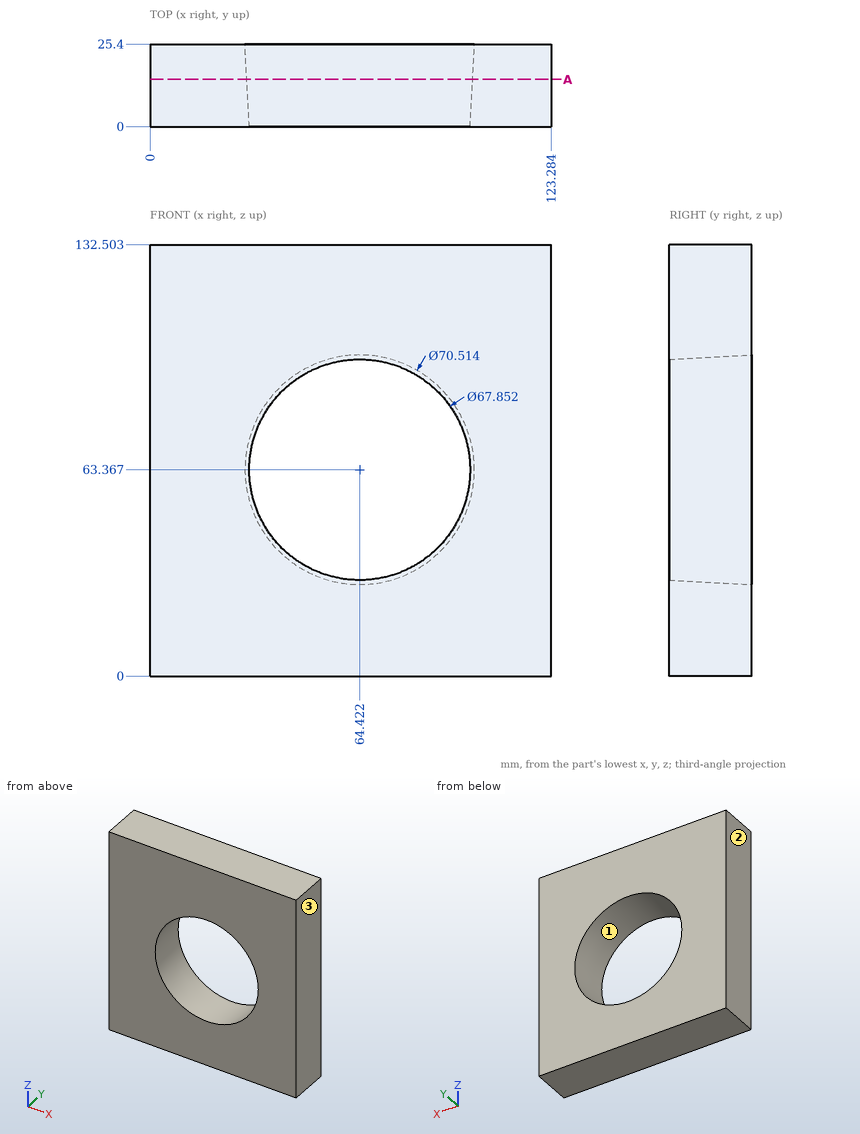
Geometry: see drawing. Coordinates: mm, zero at the bounding-box minimum. Round coordinates to 2 decimals unless told otherwise and drop trailing zeros. Write each loop counter-clockwise with the first axis right and the second up, starting at its lowest first coordinate (ties: lowest second). Pieces come first, ordered by that corner, then holes.
Item 1: Pin query (flat end, axial travel): P1, Ø3, axis at y = 13, z = 25, coming from the -X side. Return the tip coordinate at first contact, or that it passes through.
Item 2: Mould query, pull axis X, two halves, no side actions, for the marked faces 1, 2 and 3. Classes: +X half, -X half, draft (parallel to the pull), parting line (faces both ways), or undercut.
Item 3: Section query A-A (y = 14.5). Return loops of the section in (x, z) (1 decimal).
Item 4: Material intervals for L1, parallel to Z at x = 83, y = 12.5 (1 decimal); L2, parallel to Z at x = 92, y = 3.75 (1 decimal); L3, parallel to X at y = 1, z = 57 (1 decimal), sorted ascending.
Completed:
1. P1: stops at x = 0
2. face 1: undercut
2. face 2: -X half
2. face 3: +X half
3. outline: (0, 0) - (123.3, 0) - (123.3, 132.5) - (0, 132.5) - close; hole circle Ø69.4 at (64.4, 63.4)
4. L1: z = 0 to 34.2, 92.5 to 132.5
4. L2: z = 0 to 43.3, 83.5 to 132.5
4. L3: x = 0 to 31, 97.8 to 123.3
